Autodesk Inventor part; units mm, degrees
ref_plane "YZ Plane" through (0, 0, 0) normal (1, 0, 0) x (0, 1, 0)
ref_plane "XZ Plane" through (0, 0, 0) normal (0, 1, 0) x (-1, 0, 0)
ref_plane "XY Plane" through (0, 0, 0) normal (0, 0, 1) x (1, 0, 0)
sketch "Sketch1" plane through (0, 0, 0) normal (0, 1, 0) x (-1, 0, 0)
  circle A0 centre (0, 0) radius 15.875
extrude "Extrusion1" add sketch "Sketch1" along normal blind 44
sketch "Sketch2" plane through (0, 44, 0) normal (0, 1, 0) x (1, 0, 0)
  circle A0 centre (0, 0) radius 10.5
  dimension "d2" = 21
extrude "Extrusion2" add sketch "Sketch2" along normal blind 7
sketch "Sketch3" plane through (0, 51, 0) normal (0, 1, 0) x (1, 0, 0)
  circle A0 centre (0, 0) radius 3.175
extrude "Extrusion3" add sketch "Sketch3" along normal blind 23
sketch "Sketch4" plane through (0, 0, 0) normal (0, -1, 0) x (1, 0, 0)
  point P0 (0, 0)
properties part number "dc"
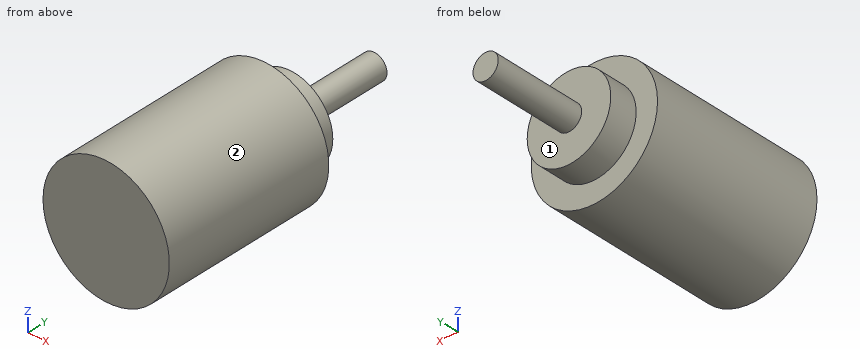
CAD build for the part. Positions are in the model's coordinates, mm. Face numbers are marked on the shaded views. A direction names the side the tool comes from. Coordinates: 2 decimals unless noted, no trailing zeros. Order: outer loops, then holes, each group sorted by start corner. A loop starts at its lowest first (then second) coordinate and runs counter-clockwise, first axis right, second up. Notation, with made-up numbers: (-28, -37.75) -> (-14, -37.75) arc R14 cw to (-14, -29.75) -> close; hole circle Ø10 at (41.5, 82). An arc over 180 degrees is marked (long way). Use one line per item in the form item = value. Start each with the question number.
1) Band-saw the part on D-D on x = 5.5. Give the cut face in (y, z), then the cut area to 3 significant figures.
2) Drill centre lines: L1, parallel to Y at x = -7.5, z = -11.5; L2, parallel to Y at x = 3, z = 9; L3, parallel to Z at x = 13, y = 24.5. Where is each one in solid material? Low to high. Write a range as [from, to].
3) Band-saw the part on A-A on x = 0. Give the cut face in (y, z) (3 decimals), then the cut area to 3 significant figures.
4) Tool access for the marked faces 1 and 2: list every direction of +Z, -Z, +X, -X, +Y, -Y with a clear straight run to the whole face (end or side of a thin tool).
5) Band-saw the part on C-C on y = 52. Give the cut face in (x, z) (3 decimals), then the cut area to 3 significant figures.
6) Drop flat-ended pins along their axis: pin 1 (8 mm diameter, centred on x = -0.5, z = 4, fed in from -Y); pin 2 (10 mm diameter, centred on y = 37.5, z = -7.5, fed in from +X); pin 3 (1 mm diameter, centred on x = 7.5, z = -1.5, fed in from +Y); pin 4 (1 mm diameter, centred on x = -5, y = 25.5, fed in from -Z). Give the stop position or say it passes through.
7) Band-saw the part on B-B on z = 0. Give the cut face in (x, y) (3 decimals), then the cut area to 3 significant figures.
Entries:
q1.outline = (0, -14.89) -> (44, -14.89) -> (44, -8.94) -> (51, -8.94) -> (51, 8.94) -> (44, 8.94) -> (44, 14.89) -> (0, 14.89) -> close
q1.area = 1,440 mm2
q2.L1 = [0, 44]
q2.L2 = [0, 51]
q2.L3 = [-9.11, 9.11]
q3.outline = (0, -15.875) -> (44, -15.875) -> (44, -10.5) -> (51, -10.5) -> (51, -3.175) -> (74, -3.175) -> (74, 3.175) -> (51, 3.175) -> (51, 10.5) -> (44, 10.5) -> (44, 15.875) -> (0, 15.875) -> close
q3.area = 1,690 mm2
q4.face_1 = +Y
q4.face_2 = +Y, -Y
q5.outline = circle Ø6.35 at (0, 0)
q5.area = 31.7 mm2
q6.pin_1 = 0
q6.pin_2 = 15.68
q6.pin_3 = 51
q6.pin_4 = -15.22
q7.outline = (-15.875, 0) -> (15.875, 0) -> (15.875, 44) -> (10.5, 44) -> (10.5, 51) -> (3.175, 51) -> (3.175, 74) -> (-3.175, 74) -> (-3.175, 51) -> (-10.5, 51) -> (-10.5, 44) -> (-15.875, 44) -> close
q7.area = 1,690 mm2
